```python
from build123d import *

# Parameters (mm, degrees)
SKETCH1_W           = 15
SKETCH1_H           = 5
BOSS_EXTRUDE1_DEPTH = 5
FILLET3_R           = 15


with BuildPart() as part:
    # Sketch1 → Boss-Extrude1 (new body)
    with BuildSketch(Plane(origin=(0, 0, 0), x_dir=(1, 0, 0), z_dir=(0, 1, 0))):
        Polygon((-26.5, -22.5), (-29.5, -22.5), (-29.5, 37.5), (-87, 37.5), (-87, 50), (-11.5, 50), (-11.5, -27.5), (-26.5, -27.5), align=None)
        with Locations((-69.5, 42.5)):
            Rectangle(SKETCH1_W, SKETCH1_H, mode=Mode.SUBTRACT)
    extrude(amount=BOSS_EXTRUDE1_DEPTH)

    # Fillet3
    fillet3_edges = [part.edges().sort_by_distance(p)[0] for p in [
        (-11.5, 2.5, -50),
    ]]
    fillet(fillet3_edges, radius=FILLET3_R)


solid = part.part
```
CAD build for the part. Positions are in the model's coordinates, mm. A direction names the side the tool comes from. Round coordinates to 2 decimals unless told otherwise and drop trailing zeros. Order: outer loops, then holes, each group sorted by start corner. A loop starts at its lowest first (then second) coordinate and runs counter-clockwise, first axis right, second up.
Q1. Slice it at A-A (x = -69). Write the cut outline in (y, z), and give its area (3 significant figures).
Q2. Slice it at B-B (y = 1.6). Write the cut outline in (x, z), and give its area (3 significant figures).
Q3. Slice it at D-D (x = -81). Write the cut outline in (y, z), and give its area (3 significant figures).
Q4. Slice it at C-C (z = 1.5). Write the cut outline in (x, y), and give its area (3 significant figures).
Q5. Drop flat-ended pins along their axis: pin 1 (2.5 mm diameter, centred on y = 3, z = -13, fed in from -X); pin 2 (1.5 mm diameter, centred on x = -27.5, y = 3.5, fed in from +Z); pin 3 (1.5 mm diameter, centred on y = 3, z = -43.5, fed in from +X). Give the stop position or say it passes through.
Q6. Which spindle directions (+Z, -Z, +X, -X, +Y, -Y) get a long thin tool onto all of the face, cutting with end or side? Do faces 1 (the flat face through (-62, 2, -42)), 2 (the flat face through (-28, 2, 22.5)), 3 (the flat face through (-19, 2, 27.5)). Say none if no direction does.
Q7. Wall check: L1, parallel to Z at x = -67.5, y = 2.9; L2, parallel to X at y = 3.1, z = 17; L3, parallel to Z at x = -52.5, y = 4.6. Give the ranges that are in metal, low to high.
Q8. Two-plate mould, pull along Z, no slides. Class faces 4 (the flat face through (-77, 2, -42)), 5 (the flat face through (-57, 2, -50)), 6 (the flat face through (-58, 2, -37.5)): pulls with the +Z half, pulls with the -Z half, needs draft (parallel to the pull), parting line crosses it, or undercut.
Results below:
1. outline: (0, -50) - (5, -50) - (5, -45) - (0, -45) - close; (0, -40) - (5, -40) - (5, -37.5) - (0, -37.5) - close
1. area: 37.5 mm2
2. outline: (-87, -50) - (-26.5, -50) arc R15 ccw to (-11.5, -35) - (-11.5, 27.5) - (-26.5, 27.5) - (-26.5, 22.5) - (-29.5, 22.5) - (-29.5, -37.5) - (-87, -37.5) - close; hole (-77, -45) - (-62, -45) - (-62, -40) - (-77, -40) - close
2. area: 1,980 mm2
3. outline: (0, -50) - (5, -50) - (5, -37.5) - (0, -37.5) - close
3. area: 62.5 mm2
4. outline: (-29.5, 0) - (-11.5, 0) - (-11.5, 5) - (-29.5, 5) - close
4. area: 90.0 mm2
5. pin 1: stops at x = -29.5
5. pin 2: stops at z = 22.5
5. pin 3: stops at x = -13.66
6. face 1: +Y, -Y
6. face 2: +Z, -X, +Y, -Y
6. face 3: +Z, +X, -X, +Y, -Y
7. L1: z = -50 to -45, -40 to -37.5
7. L2: x = -29.5 to -11.5
7. L3: z = -50 to -37.5
8. face 4: undercut
8. face 5: pulls with the -Z half
8. face 6: pulls with the +Z half
